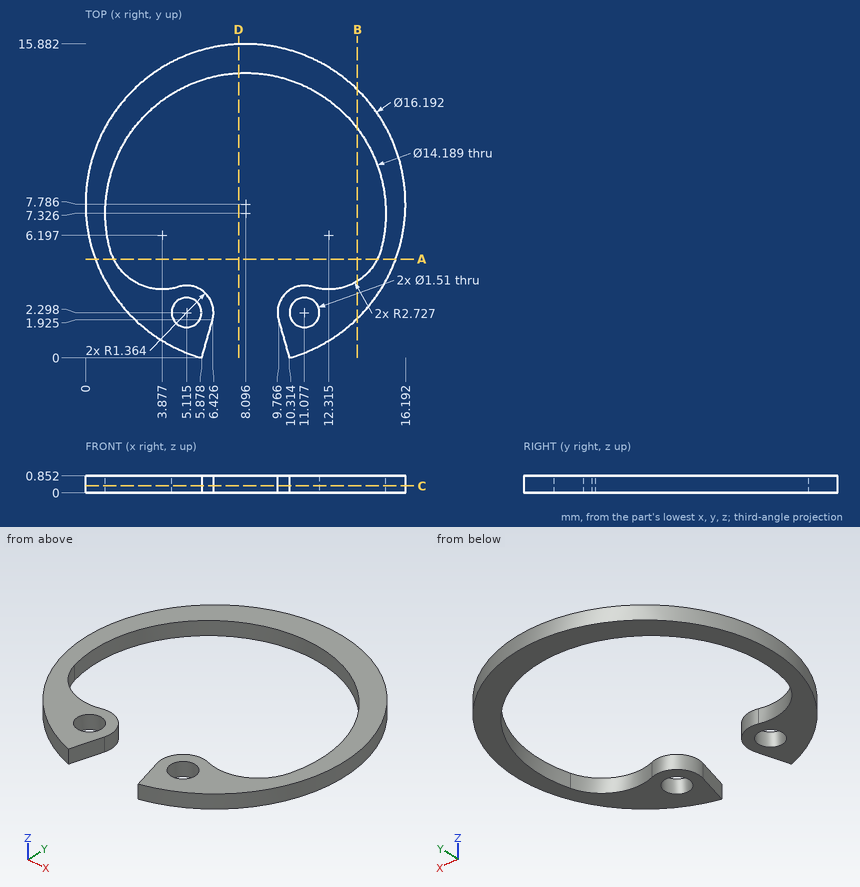
Study the drawing (mm; zero at the part's minimum x, y, z) and answer. Coordinates: 2 decimals unless noted, no trailing zeros. Write each loop counter-clockwise with the first axis right and the second up, starting at its lowest first coordinate (ties: lowest second). Pieces come first, ordered by that corner, then holes. Notation, with made-up numbers: M 23,60 L 27,60 A16 ccw 27,89 Z; hole C 17,37.5 d4. An arc over 180 degrees is marked long. Use a Markdown table: item, result. Add a question column.
1. Section D-D (x = 7.75) is taken. Give the vertices of the cut face in (y, z) (1 decimal).
2. Section B-B (x = 13.75) is taken. Give the vertices of the cut face in (y, z).
3. Section C-C (z = 0.35) is taken. Count the separate pieces of the cut face and the enclosed holes in it.
4. Section A-A (y = 5) is taken. Give the vertices of the cut face in (x, z) (1 decimal).
5. Given P1, Ø1.2, axis at x = 11.08, y = 2.3, coming from the +Z side, flat-ended and moving along its own axis, determine where the tip first touches the part or whether it passes through.
6. Straight lines are drawn through the part: line 1 along Y through (x, z) = (10.75, 0.8) (1 decimal); line 2 along Y through (x, z) = (5.75, 0.7) (1 decimal); line 3 along X through (y, z) = (7, 0.1). For each, find the intervals that lie inside material, in ascending order. Write a range as [from, to].
Data:
| question | item | result |
|---|---|---|
| 1 | outline | M 14.4,0 L 15.9,0 L 15.9,0.9 L 14.4,0.9 Z |
| 2 | outline | M 1.99,0 L 3.88,0 L 3.88,0.85 L 1.99,0.85 Z; M 11.61,0 L 13.58,0 L 13.58,0.85 L 11.61,0.85 Z |
| 3 | separate pieces | 1 |
| 3 | enclosed holes | 2 |
| 4 | outline | M 0.5,0 L 1.4,0 L 1.4,0.9 L 0.5,0.9 Z; M 14.8,0 L 15.7,0 L 15.7,0.9 L 14.8,0.9 Z |
| 5 | P1 | passes through |
| 6 | line 1 | y = [0.1, 1.6], [3, 3.6], [13.9, 15.4] |
| 6 | line 2 | y = [0, 1.9], [2.7, 3.5], [14, 15.5] |
| 6 | line 3 | x = [0.04, 1.01], [15.18, 16.15] |
